Geometry: final body of the model. Coordinates: model frame, mm. Face numbers are marked on the shaded views. A direction names the side the tool comes from. Give positions to 0.01 mm unless a question says otherwise; leave off trailing zeros. Loops run counter-clockwise (first coordinate to the right, second up) from the corner with the lowest first, then second, coordinate; pieces in that order, holes last.
1. Section C-C, the plane y = -76.5. Output: boundary loops of the cut face in (x, z).
2. Section B-B, the plane x = 0. Output: boundary loops of the cut face in (y, z).
3. Section A-A, the plane z = 0. Output: boundary loops of the cut face in (x, y).
4. Material intervals for line 1 along Y through (x, z) = (-0.75, 10.5); line 2 along Z through (x, y) = (0, -6.5); line 3 along X through (y, z) = (-29, 0.5), sorted ascending.
5. Access query for the marked faces 1, 2 and 3. Directions: +Z, -Z, +X, -X, +Y, -Y. A direction counts if a zero-diameter tool reaches every point of the face in a straight line with its end or side. Return the directions, or none.
6. First-contact query: P1, Ø2.5, axis at y = -12.5, z = 7.5, coming from the +X side; P2, Ø1, axis at x = 1.5, y = -64, coming from the +Z side; P3, Ø1.5, axis at y = -13.5, z = 8.5, coming from the -X side. Flat tips, straight axial feed; report the tip coordinate or a pass-through.
7. Section D-D, the plane y = -36.5. Output: boundary loops of the cut face in (x, z), then the cut area to 3 significant figures.
from build123d import *

# Parameters (mm, degrees)
CHAMFER_1_SIZE      = 1
CUT_EXTRUDE_1_DEPTH = 6
CHAMFER_2_SIZE      = 1


with BuildPart() as part:
    # 草图1 → 旋转1 (revolve)
    with BuildSketch(Plane.XY):
        Polygon((0, 0), (10, 0), (10, -45), (11.5, -45), (11.5, -100), (7.5, -100), (7.5, -110), (0, -110), align=None)
    revolve(axis=Axis((0, -110, 0), (0, 1, 0)))

    # 倒角1
    chamfer_1_edges = [part.edges().sort_by_distance(p)[0] for p in [
        (-10, 0, 0),
    ]]
    chamfer(chamfer_1_edges, length=CHAMFER_1_SIZE)

    # 草图2 → 切除-拉伸1 (cut, through all)
    with BuildSketch(Plane.XY.offset(6.5)):
        with BuildLine():
            Line((3, -5), (3, -25))
            ThreePointArc((3, -25), (0, -28), (-3, -25))
            Line((-3, -25), (-3, -5))
            ThreePointArc((-3, -5), (0, -2), (3, -5))
        make_face()
    extrude(amount=CUT_EXTRUDE_1_DEPTH, mode=Mode.SUBTRACT)

    # 倒角2
    chamfer_2_edges = [part.edges().sort_by_distance(p)[0] for p in [
        (-7.5, -110, 0),
    ]]
    chamfer(chamfer_2_edges, length=CHAMFER_2_SIZE)


solid = part.part
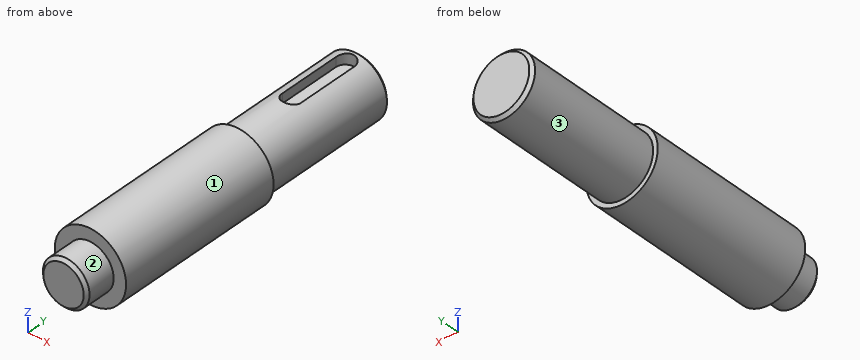
Answers below:
1. outline: circle Ø23 at (0, 0)
2. outline: (-110, -6.5) - (-109, -7.5) - (-100, -7.5) - (-100, -11.5) - (-45, -11.5) - (-45, -10) - (-1, -10) - (0, -9) - (0, 9) - (-1, 10) - (-2, 10) - (-2, 6.5) - (-28, 6.5) - (-28, 10) - (-45, 10) - (-45, 11.5) - (-100, 11.5) - (-100, 7.5) - (-109, 7.5) - (-110, 6.5) - close
3. outline: (-11.5, -100) - (-7.5, -100) - (-7.5, -109) - (-6.5, -110) - (6.5, -110) - (7.5, -109) - (7.5, -100) - (11.5, -100) - (11.5, -45) - (10, -45) - (10, -1) - (9, 0) - (-9, 0) - (-10, -1) - (-10, -45) - (-11.5, -45) - close
4. line 1: y = -100 to -45
4. line 2: z = -10 to 6.5
4. line 3: x = -9.99 to 9.99
5. face 1: +Y, -Y
5. face 2: -Y
5. face 3: +Y
6. P1: stops at x = 7.81
6. P2: stops at z = 11.46
6. P3: stops at x = -6.32
7. outline: circle Ø20 at (0, 0)
7. area: 314 mm2
